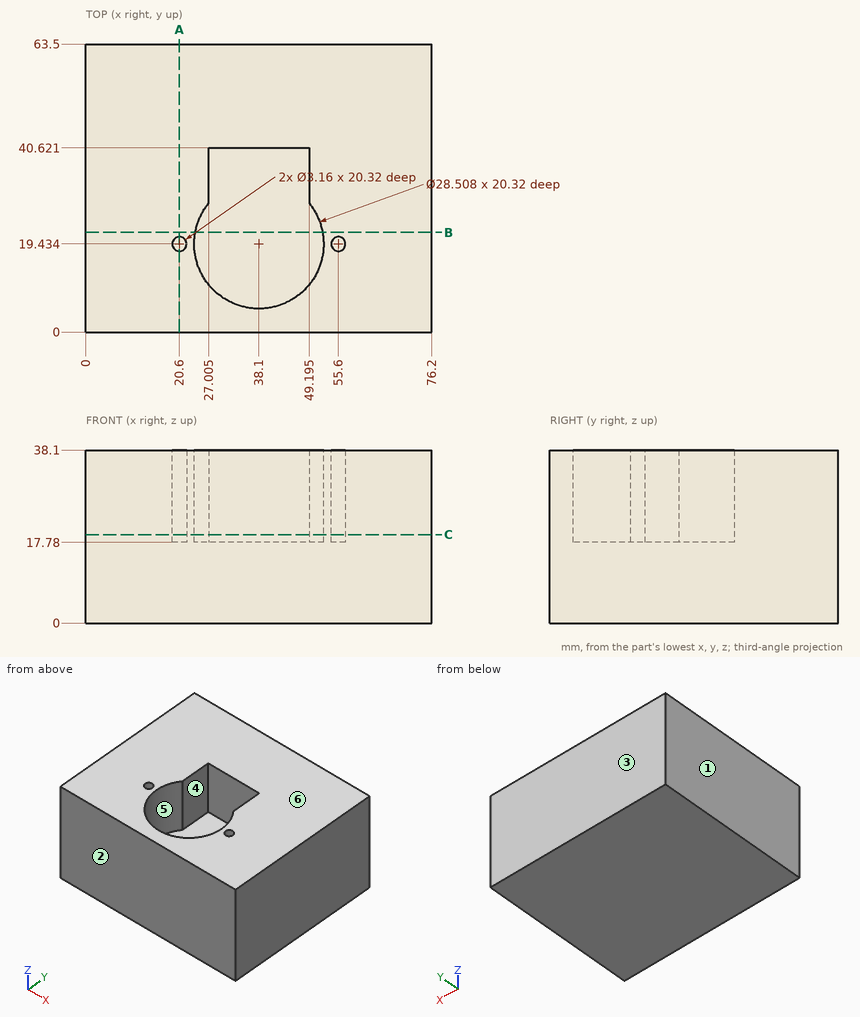
Part print with two shaded views. Sizes in mm from the minimum x, y, z corner. A direction names the side the tool comes from. Coordinates: 2 decimals unless noted, no trailing zeros. Write each loop counter-clockwise with the first axis right and the second up, starting at its lowest first coordinate (ties: lowest second). Pieces come first, ordered by that corner, then holes. Notation, with made-up numbers: (-28.75, 35) - (25.25, 35) arc R24 ccw to (25.25, 73) - close; hole circle Ø8 at (-31, 87). An arc over 180 degrees is marked (long way). Put each result on its own line as item: value.
1. Flat gauge pin, fed straight in: pin 1 Ø8.5 at (x, y) = (32, 22.5) entering from +Z. Where does the tip first touch, or does it go through?
Final values:
pin 1: stops at z = 17.78
2. Band-saw the part on A-A (x = 20.6). Write the cut outline in (y, z) (1 decimal), then the cut area to 4 significant figures.
Final values:
outline: (0, 0) - (63.5, 0) - (63.5, 38.1) - (21, 38.1) - (21, 17.8) - (17.9, 17.8) - (17.9, 38.1) - (0, 38.1) - close
area: 2,355 mm²
3. Two-plate mould, pull along Y, no slides. Class the marked faces 1, 2, 3 and 4: +Y half, -Y half, draft (parallel to the pull), parting line (faces both ways), or undercut.
Final values:
face 1: draft
face 2: -Y half
face 3: +Y half
face 4: undercut
4. 3-axis set-ups, long thin cutter, end or side, ignore diameter. For the marked faces 5 and 6: which of +Z, -Z, +X, -X, +Y, -Y reach the whole face in a straight line?
Final values:
face 5: +Z
face 6: +Z, +X, -X, +Y, -Y
5. Probe line 1 along Y through (x, z) = (20.6, 30.5) (1 decimal); line 2 along X through (y, z) = (28.5, 20.5) (1 decimal); line 3 along Z through (x, y) = (26.5, 14). List the from-to ranges inside material, lowest first. Write a range as [from, to].
Final values:
line 1: y = [0, 17.9], [21, 63.5]
line 2: x = [0, 27], [49.2, 76.2]
line 3: z = [0, 17.78]
6. Band-saw the part on B-B (y = 22). Write the cut outline in (x, z).
Final values:
outline: (0, 0) - (76.2, 0) - (76.2, 38.1) - (52.12, 38.1) - (52.12, 17.78) - (24.08, 17.78) - (24.08, 38.1) - (0, 38.1) - close
7. Band-saw the part on C-C (z = 19.5). Write the cut outline in (x, y) (1 decimal), then the cut area to 4 significant figures.
Final values:
outline: (0, 0) - (76.2, 0) - (76.2, 63.5) - (0, 63.5) - close; hole circle Ø3.2 at (20.6, 19.4); hole (27, 28.4) arc R14.3 ccw (long way) to (49.2, 28.4) - (49.2, 40.6) - (27, 40.6) - close; hole circle Ø3.2 at (55.6, 19.4)
area: 3,995 mm²
